Here's the drawing with two shaded views (mm, measured from the low corner). I have some questions. Round coordinates to 2 decimals unless told otherwise and drop trailing zeros. Order: outer loops, then holes, each group sorted by start corner. A loop starts at its lowest first (then second) coordinate and runs counter-clockwise, first axis right, second up.
Q1. If we section it at C-C (y = 5.75): Please give me the cut outline in (x, z), plus the area to 3 significant figures.
Q2. If we section it at B-B (z = 3): Please give me the cut outline in (x, y).
Q3. If I drill on line 1 (X direction, y = 1, z = 5); line 2 (X direction, y = 5.25, z = 5.08); line 3 (Z direction, x = 4.25, y = 1.75), over which ranges is the centre line in solid material (lowest first)?
Q4. If we section it at A-A (x = 5.08): Please give me the cut outline in (y, z).
Q5. If we section it at D-D (y = 2.25): Please give me the cut outline in (x, z), plus the area to 3 significant figures.
Q6. We'd pull the mould along Z, two halves only. Please class the marked faces 1, 2, 3 and 4: pulls with the +Z half, pulls with the -Z half, needs draft (parallel to the pull), parting line crosses it, or undercut.
Q7. Will these pins go through, and if not, where does the flat tip stop? P1, Ø1.5, axis at x = 4, z = 5.5, coming from the -Y side; P2, Ø1.1, axis at y = 1.5, z = 4, coming from the +X side; P3, Ø3, axis at x = 7, y = 5.5, coming from the +Z side; P4, Ø2, axis at x = 9, y = 3.5, coming from the -Z side.
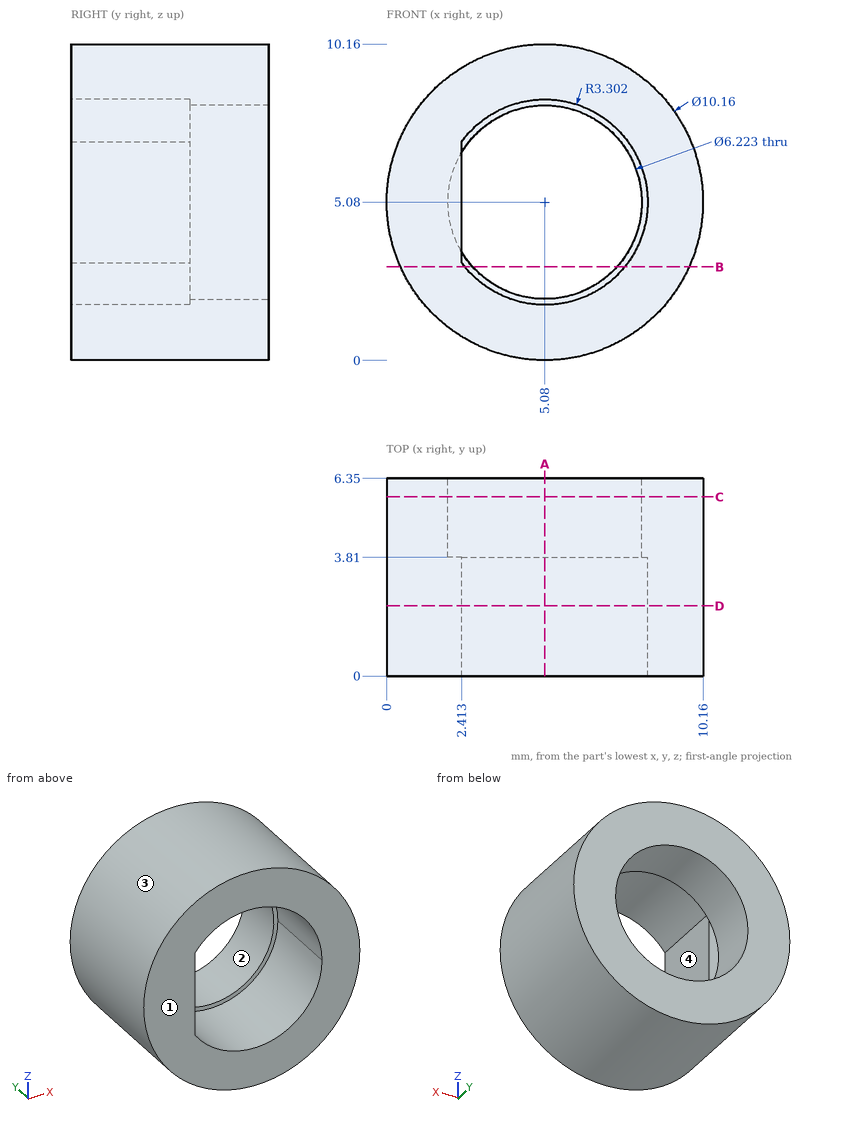
Solution:
1. outline: circle Ø10.16 at (5.08, 5.08); hole circle Ø6.22 at (5.08, 5.08)
1. area: 50.7 mm2
2. outline: (0.45, 0) - (2.52, 0) - (2.52, 3.81) - (2.77, 3.81) - (2.77, 6.35) - (0.45, 6.35) - close; (7.39, 3.81) - (7.64, 3.81) - (7.64, 0) - (9.71, 0) - (9.71, 6.35) - (7.39, 6.35) - close
3. line 1: x = 0 to 2.41, 8.38 to 10.16
3. line 2: x = 0 to 1.97, 8.19 to 10.16
3. line 3: z = 0.07 to 1.88, 8.28 to 10.09
4. outline: (0, 0) - (6.35, 0) - (6.35, 1.97) - (3.81, 1.97) - (3.81, 1.78) - (0, 1.78) - close; (0, 8.38) - (3.81, 8.38) - (3.81, 8.19) - (6.35, 8.19) - (6.35, 10.16) - (0, 10.16) - close
5. outline: circle Ø10.16 at (5.08, 5.08); hole (2.41, 3.13) arc R3.3 ccw (long way) to (2.41, 7.03) - close
5. area: 48.5 mm2
6. face 1: needs draft
6. face 2: undercut
6. face 3: parting line crosses it
6. face 4: undercut
7. P1: passes through
7. P2: stops at x = 10.13
7. P3: stops at z = 10.14
7. P4: stops at z = 0.92
